```python
from build123d import *

# Parameters (mm, degrees)
BOSS_EXTRUDE1_DEPTH = 23
BOSS_EXTRUDE2_DEPTH = 54
SKETCH5_R           = 4
CUT_EXTRUDE1_DEPTH  = 52
CUT_EXTRUDE5_DEPTH  = 133.527415876
SKETCH8_R           = 6
CUT_EXTRUDE6_DEPTH  = 127.3759431
CUT_EXTRUDE7_DEPTH  = 120.427295851
SKETCH10_W          = 28
SKETCH10_H          = 28
CUT_EXTRUDE8_DEPTH  = 10
CHAMFER1_SIZE       = 2
CHAMFER2_SIZE       = 1


with BuildPart() as part:
    # Sketch1 → Boss-Extrude1 (new, symmetric)
    with BuildSketch(Plane.XY):
        Polygon((104, 0), (97.5, 0), (97.5, 2), (-97.5, 2), (-97.5, 0), (-104, 0), (-99.985564599, 14), (99.985564599, 14), align=None)
    extrude(amount=BOSS_EXTRUDE1_DEPTH, both=True)

    # Sketch3 → Boss-Extrude2 (add)
    with BuildSketch(Plane(origin=(0, 14, 0), x_dir=(1, 0, 0), z_dir=(0, 1, 0))):
        with BuildLine():
            Line((-48.837700706, 23.040811394), (48.837700706, 23.040811394))
            ThreePointArc((48.837700706, 23.040811394), (54, 0), (48.837700706, -23.040811394))
            Line((48.837700706, -23.040811394), (-48.837700706, -23.040811394))
            ThreePointArc((-48.837700706, -23.040811394), (-54, 0), (-48.837700706, 23.040811394))
        make_face()
    extrude(amount=BOSS_EXTRUDE2_DEPTH)

    # Sketch5 → Cut-Extrude1 (cut)
    with BuildSketch(Plane(origin=(0, 68, 0), x_dir=(1, 0, 0), z_dir=(0, 1, 0))):
        with Locations(Location((0, 0, 0), (0, 0, 180))):
            Circle(SKETCH5_R)
    extrude(amount=-CUT_EXTRUDE1_DEPTH, mode=Mode.SUBTRACT)

    # Sketch6 → Cut-Extrude5 (cut, through all)
    with BuildSketch(Plane.XY.offset(23.040811394)):
        with BuildLine():
            Line((-28, 374.971379092), (-28, 68))
            Line((-28, 68), (-28, 52))
            Line((-28, 52), (-23.664319132, 52))
            ThreePointArc((-23.664319132, 52), (0, 24), (23.664319132, 52))
            Line((23.664319132, 52), (28, 52))
            Line((28, 52), (28, 68))
            Line((28, 68), (28, 374.971379092))
            Line((28, 374.971379092), (28, 988.914137277))
            Line((28, 988.914137277), (-28, 988.914137277))
            Line((-28, 988.914137277), (-28, 374.971379092))
        make_face()
    extrude(amount=-CUT_EXTRUDE5_DEPTH, mode=Mode.SUBTRACT)

    # Sketch8 → Cut-Extrude6 (cut, through all)
    with BuildSketch(Plane(origin=(0, 68, 0), x_dir=(1, 0, 0), z_dir=(0, 1, 0))):
        with Locations(Location((-39, 0.040811394, 0), (0, 0, 180))):
            Circle(SKETCH8_R)
        with Locations(Location((39, 0.040811394, 0), (0, 0, 180))):
            Circle(SKETCH8_R)
    extrude(amount=-CUT_EXTRUDE6_DEPTH, mode=Mode.SUBTRACT)

    # Sketch9 → Cut-Extrude7 (cut, through all)
    with BuildSketch(Plane(origin=(0, 14, 0), x_dir=(1, 0, 0), z_dir=(0, 1, 0))):
        with BuildLine():
            Line((-85, 6), (-77, 6))
            ThreePointArc((-77, 6), (-71, 0), (-77, -6))
            Line((-77, -6), (-85, -6))
            ThreePointArc((-85, -6), (-91, 0), (-85, 6))
        make_face()
        with BuildLine():
            Line((85, 6), (77, 6))
            ThreePointArc((77, 6), (71, 0), (77, -6))
            Line((77, -6), (85, -6))
            ThreePointArc((85, -6), (91, 0), (85, 6))
        make_face()
    extrude(amount=-CUT_EXTRUDE7_DEPTH, mode=Mode.SUBTRACT)

    # Sketch10 → Cut-Extrude8 (cut)
    with BuildSketch(Plane(origin=(0, 2, 0), x_dir=(-1, 0, 0), z_dir=(0, -1, 0))):
        with Locations((39, 0.040811394)):
            Rectangle(SKETCH10_W, SKETCH10_H)
        with Locations((-39, 0.040811394)):
            Rectangle(SKETCH10_W, SKETCH10_H)
    extrude(amount=-CUT_EXTRUDE8_DEPTH, mode=Mode.SUBTRACT)

    # Chamfer1
    chamfer1_edges = [part.edges().sort_by_distance(p)[0] for p in [
        (0, 24, -23.040811394),
        (0, 24, 23.040811394),
    ]]
    chamfer(chamfer1_edges, length=CHAMFER1_SIZE)

    # Chamfer2
    chamfer2_edges = [part.edges().sort_by_distance(p)[0] for p in [
        (91, 14, 0),
        (81, 14, -6),
        (71, 14, 0),
        (81, 14, 6),
        (-91, 14, 0),
        (-81, 14, 6),
        (-71, 14, 0),
        (-81, 14, -6),
    ]]
    chamfer(chamfer2_edges, length=CHAMFER2_SIZE)


solid = part.part
```
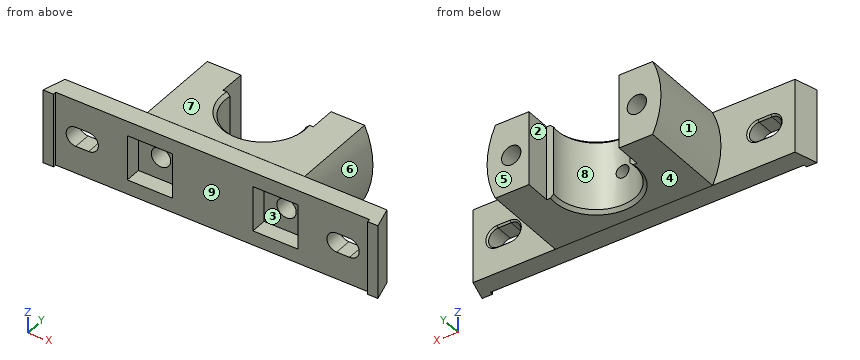
CAD build for the part. Positions are in the model's coordinates, mm. Face numbers are marked on the shaded views. A direction names the side the tool comes from. Round coordinates to 2 decimals unless told otherwise and drop trailing zeros. Order: outer loops, then holes, each group sorted by start corner. A loop starts at its lowest first (then second) coordinate and runs counter-clockwise, first axis right, second up. Notation, with made-up numbers: (6, 75) -> (48, 75) arc R19 cw to (48, 107) -> close; hole circle Ø11 at (31, 49.5). An arc over 180 degrees is marked (long way). One line per question, with ' | ' between items.
Q1. Which spindle directions (+Z, -Z, +X, -X, +Y, -Y) get a long thin tool onto all of the face, cutting with end or side? Do the marked faces 1, 2, 3, 4 and 5. Say none if no direction does.
Completed:
face 1: -X, +Y | face 2: +Z, -Z, +Y | face 3: -Y | face 4: -Z, +X, -X, +Y, -Y | face 5: +Z, -Z, +X, -X, +Y
Q2. Slice it at D-D (z = 16). Write the cut outline in (x, y), then the cut area to 3 significant figures.
Completed:
outline: (-104, 0) -> (-97.5, 0) -> (-97.5, 2) -> (97.5, 2) -> (97.5, 0) -> (104, 0) -> (99.99, 14) -> (51.58, 14) -> (51.58, 68) -> (28, 68) -> (28, 52) -> (23.66, 52) arc R24 cw (long way) to (-23.66, 52) -> (-28, 52) -> (-28, 68) -> (-51.58, 68) -> (-51.58, 14) -> (-99.99, 14) -> close | area: 6,040 mm^2
Q3. Slice it at B-B (y = 61). Write the cut outline in (x, z).
Completed:
outline: (-48.84, -23.04) -> (-28, -23.04) -> (-28, 23.04) -> (-48.84, 23.04) arc R54 ccw to start; (28, -23.04) -> (48.84, -23.04) arc R54 ccw to (48.84, 23.04) -> (28, 23.04) -> close; hole circle Ø12 at (-39, -0.04); hole circle Ø12 at (39, -0.04)
Q4. Drop flat-ended pins along their axis: pin 1 (8 mm diameter, centred on x = 37.5, y = 6, fed in from -Z); pin 2 (2 mm diameter, centred on y = 13, z = 7.5, fed in from +X); pin 3 (13 mm diameter, centred on y = 57, z = -10.5, fed in from -X). Give the stop position or say it passes through.
Completed:
pin 1: stops at z = -23 | pin 2: stops at x = 100.56 | pin 3: stops at x = -53.85
Q5. Two-plate mould, pull along X, no slides. Class the marked faces 6, 7, 8 and 9: released by +X, released by -X, zero draft, split by the parting line, or undercut.
Completed:
face 6: released by +X | face 7: zero draft | face 8: undercut | face 9: undercut
Q6. Slice it at C-C (x = 0). Write the cut outline in (y, z).
Completed:
outline: (2, -23) -> (14, -23) -> (14, -23.04) -> (22, -23.04) -> (24, -21.04) -> (24, -4) -> (16, -4) -> (16, 4) -> (24, 4) -> (24, 21.04) -> (22, 23.04) -> (14, 23.04) -> (14, 23) -> (2, 23) -> close
Q7. Probe probe 1 along X at (y, z) = (48, 4.5); probe 2 along Z at (x, y) = (0, 20.75); probe 3 along X at (y, z) = (23, -2). List the from-to ranges inside material, lowest first.
Completed:
probe 1: x = -53.81 to -42.92, -35.08 to -24, 24 to 35.08, 42.92 to 53.81 | probe 2: z = -23.04 to -4, 4 to 23.04 | probe 3: x = -53.96 to -44.67, -33.33 to -3.46, 3.46 to 33.33, 44.67 to 53.96
Q8. Slice it at A-A (x = 39). Write the cut outline in (y, z), then the cut area to 3 significant figures.
Completed:
outline: (2, -23) -> (14, -23) -> (14, -23.04) -> (68, -23.04) -> (68, -6.04) -> (12, -6.04) -> (12, -14.04) -> (2, -14.04) -> close; (2, 13.96) -> (12, 13.96) -> (12, 5.96) -> (68, 5.96) -> (68, 23.04) -> (14, 23.04) -> (14, 23) -> (2, 23) -> close | area: 2,090 mm^2
